```python
from build123d import *

# Parameters (mm, degrees)
F0_W     = 18.651318
F0_H     = 71.940791
F2_R     = 15.850572
F3_DEPTH = 78
F4_R     = 10.510911
F5_DEPTH = 80


with BuildPart() as f1:
    # F0 (on Front) → F1 (revolve)
    with BuildSketch(Plane.XZ):
        with Locations((42.335527, -0.592103)):
            Rectangle(F0_W, F0_H)
    revolve(axis=Axis((0, 0, 7.253291), (0, 0, -1)))

    # F2 (on Right) → F3 (join)
    with BuildSketch(Plane.YZ):
        Circle(F2_R)
    extrude(amount=F3_DEPTH)

    # F4 (on Right) → F5 (cut)
    with BuildSketch(Plane.YZ):
        Circle(F4_R)
    extrude(amount=F5_DEPTH, mode=Mode.SUBTRACT)


solid = f1.part
```
For this review, take the finished solid that the model builds, in its own axes (mm). A direction names the side the tool comes from. Coordinates: 2 decimals unless noted, no trailing zeros. Write each loop counter-clockwise with the first axis right and the second up, starting at its lowest first coordinate (ties: lowest second). Pieces come first, ordered by that corner, then holes. Notation, with made-up numbers: (33.25, 57.5) -> (78.25, 57.5) arc R26 cw to (78.25, 79.5) -> close; hole circle Ø5 at (46, 28.25). An arc over 180 degrees is marked (long way). Put each result on its own line as item: value.
Q1. The part is to be moulded in two halves that separate along X. For faces 4 (the flat face through (1, 34, 35.378)), 5 (the flat face through (78, 10.3, -3.3)), 6 (the cylindrical face through (16.274, 14.642, -6.071)), 7 (the cylindrical face through (-40.997, 31.435, -0.089)), say which applies: +X half, -X half, draft (parallel to the pull), parting line (faces both ways), or undercut.
From the geometry:
face 4: draft
face 5: +X half
face 6: undercut
face 7: parting line
Q2. Take a section at C-C, the plane y = -27.5. State the section outline as (x, z) points.
From the geometry:
outline: (-43.73, -36.56) -> (-18.26, -36.56) -> (-18.26, 35.38) -> (-43.73, 35.38) -> close; (18.26, -36.56) -> (43.73, -36.56) -> (43.73, 35.38) -> (18.26, 35.38) -> close
Q3. Take a section at B-B, the plane z = 24.5. State the section outline as (x, y) points, then the cut area to 3 significant figures.
From the geometry:
outline: circle Ø103.32 at (0, 0); hole circle Ø66.02 at (0, 0)
area: 4,960 mm2
Q4. Take a section at A-A, the plane y = 0. State the section outline as (x, z) points.
From the geometry:
outline: (-51.66, -36.56) -> (-33.01, -36.56) -> (-33.01, 35.38) -> (-51.66, 35.38) -> close; (0, -15.85) -> (33.01, -15.85) -> (33.01, -36.56) -> (51.66, -36.56) -> (51.66, -15.85) -> (78, -15.85) -> (78, -10.51) -> (0, -10.51) -> close; (0, 10.51) -> (78, 10.51) -> (78, 15.85) -> (51.66, 15.85) -> (51.66, 35.38) -> (33.01, 35.38) -> (33.01, 15.85) -> (0, 15.85) -> close
Q5. Tool access review of faces 1 (the flat face through (1, 34, -36.562)), 2 (the flat face through (0, 10.3, -3.3)), 3 (the cylindrical face through (63.383, -15.835, 0.697)): name each direction out of +Z, -Z, +X, -X, +Y, -Y from which nothing blocks a thin tool from reaching the whole face with its end or side.
From the geometry:
face 1: -Z, +X, -X, +Y, -Y
face 2: +Z, -Z
face 3: +X
Q6. Take a section at D-D, the plane x = -7.5. State the section outline as (y, z) points.
From the geometry:
outline: (-51.11, -36.56) -> (-32.15, -36.56) -> (-32.15, 35.38) -> (-51.11, 35.38) -> close; (32.15, -36.56) -> (51.11, -36.56) -> (51.11, 35.38) -> (32.15, 35.38) -> close
Q7. Wall thickness on L1, parallel to Y at x = 0, z = -18; L2, parallel to Y at x = 19.5, z = -11; L3, parallel to Y at x = 22, z = 0: over which ranges is each line inside the solid? List them lowest first.
From the geometry:
L1: y = -51.66 to -33.01, 33.01 to 51.66
L2: y = -47.84 to -26.63, -11.41 to 11.41, 26.63 to 47.84
L3: y = -46.74 to -24.61, -15.85 to -10.51, 10.51 to 15.85, 24.61 to 46.74
Q8. Clearance check with flat-ended pins moving along their axes: pin 1 Ø6 at (x, z) = (-8, 26) entering from -Y; pin 2 Ø5 at (x, y) = (8, 18.5) entering from +Z; pin 3 Ø4 at (x, z) = (8, -23.5) entering from +Y; pin 4 Ø1.5 at (x, z) = (-32, 13.5) entering from +Y. State where each tip first meets the part, or that it passes through.
From the geometry:
pin 1: stops at y = -51.42
pin 2: passes through
pin 3: stops at y = 51.31
pin 4: stops at y = 41.14
